Geometry check sheet. Reference: the model listing, model coordinates, mm. A direction names the side the tool comes from. Coordinates: 2 decimals unless noted, no trailing zeros. Loops run counter-clockwise (first coordinate to the right, second up) from the corner with the lowest first, then second, coordinate; pieces in that order, holes last. Notation, with made-up numbers: (-11, 73.25) - (29, 73.25) arc R32 cw to (29, 105.25) - close; hole circle Ø9 at (47.25, 60.25). An arc over 180 degrees is marked (long way). Write item = value, one per line. Start each with the question number.
from build123d import *

# Parameters (mm, degrees)
SKETCH2_W           = 200
SKETCH2_H           = 200
BOSS_EXTRUDE1_DEPTH = 50
SHELL1_T            = -20
CUT_EXTRUDE1_DEPTH  = 50
SKETCH5_R           = 50
BOSS_EXTRUDE2_DEPTH = 28
SKETCH6_R           = 40
CUT_EXTRUDE2_DEPTH  = 34
SKETCH7_R           = 14
CUT_EXTRUDE4_DEPTH  = 46


with BuildPart() as part:
    # Sketch2 → Boss-Extrude1 (new body)
    with BuildSketch(Plane.XY):
        with Locations((-40.678946788, -125.067928938)):
            Rectangle(SKETCH2_W, SKETCH2_H)
    extrude(amount=-BOSS_EXTRUDE1_DEPTH)

    # Shell1
    shell1_openings = [part.faces().sort_by_distance(p)[0] for p in [
        (-40.678946788, -125.067928938, -50),
    ]]
    offset(amount=SHELL1_T, openings=shell1_openings, kind=Kind.INTERSECTION)

    # Sketch3 → Cut-Extrude1 (cut)
    with BuildSketch(Plane.XY):
        Polygon((-13.228603608, -25.067928938), (1.821053212, -51.157579637), (-83.178946788, -51.157579637), (-68.129289968, -25.067928938), align=None)
    extrude(amount=-CUT_EXTRUDE1_DEPTH, mode=Mode.SUBTRACT)

    # Sketch5 → Boss-Extrude2 (add)
    with BuildSketch(Plane(origin=(0, 0, -20), x_dir=(-1, 0, 0), z_dir=(0, 0, -1))):
        with Locations((40.678946788, -125.067928938)):
            Circle(SKETCH5_R)
    extrude(amount=BOSS_EXTRUDE2_DEPTH)

    # Sketch6 → Cut-Extrude2 (cut)
    with BuildSketch(Plane.XY):
        with Locations((-40.678946788, -125.067928938)):
            Circle(SKETCH6_R)
    extrude(amount=-CUT_EXTRUDE2_DEPTH, mode=Mode.SUBTRACT)

    # Sketch7 → Cut-Extrude4 (cut)
    with BuildSketch(Plane(origin=(0, -45.067928938, 0), x_dir=(-1, 0, 0), z_dir=(0, -1, 0))):
        with Locations(Location((40.678946788, 32, 0), (0, 0, 301.002719134))):
            Circle(SKETCH7_R)
    extrude(amount=CUT_EXTRUDE4_DEPTH, mode=Mode.SUBTRACT)


solid = part.part
(1) Sectioned sample at C-C on z = -10.5. Enter the section's corners in (x, y), plus the area to 3 significant figures.
(2) Draft check along Y on faces 5 (the face through (-105, -25.068, -25)), 6 (the face through (-49, -206, -50)), 7 (the face through (-42, -205.068, -35)). Enter one of: pulls with the +Y half, pulls with the -Y half, needs draft (parallel to the pull), parting line crosses it, or undercut.
(3) Sectioned sample at B-B on x = 30.5. Enter the section's corners in (y, z), plus the area to 3 significant figures.
(4) Scan lines: line 1 (Y direction, x = 27.5, z = -30); line 2 (X direction, y = -190.5, z = -42); line 3 (Y direction, x = -69, z = -31). Record each from-to range of solid material in increasing order.
(5) Sectioned sample at A-A on z = -28.5. Enter the section's corners in (x, y).
(6) Sectioned sample at D-D on y = -147. Enter the section's corners in (x, z), plus the area to 3 significant figures.
(7) Depth check by flat-ended pin: pin 1 (10 mm diameter, centred on x = -108, y = -173, fed in from +Z); pin 2 (9.5 mm diameter, centred on x = -38.5, z = -41.5, fed in from +Y). Enter the tip coordinate at first touch or a pass-through.
(8) Tool access check on faces 1 (the face through (-22.221, -160.555, -16.762)), 2 (the face through (39.321, -126, -35)), 3 (the face through (-40, -51.158, -10)), 4 (the face through (-41, -91.068, -40)). Record the directions out of +Z, -Z, +X, -X, +Y, -Y that give a thin tool (end or side, any length) a straight path to the whole face; none if there is none.
Working result:
q1.outline = (-140.68, -225.07) - (59.32, -225.07) - (59.32, -25.07) - (-13.23, -25.07) - (1.82, -51.16) - (-83.18, -51.16) - (-68.13, -25.07) - (-140.68, -25.07) - close; hole circle Ø80 at (-40.68, -125.07)
q1.area = 33,100 mm2
q2.face_5 = pulls with the +Y half
q2.face_6 = needs draft
q2.face_7 = undercut
q3.outline = (-225.07, -50) - (-205.07, -50) - (-205.07, -20) - (-45.07, -20) - (-45.07, -50) - (-25.07, -50) - (-25.07, 0) - (-225.07, 0) - close
q3.area = 5,200 mm2
q4.line_1 = -225.07 to -205.07, -45.07 to -25.07
q4.line_2 = -140.68 to -120.68, 39.32 to 59.32
q4.line_3 = -225.07 to -205.07, -166.27 to -153.32, -96.82 to -83.86, -26.58 to -25.07
q5.outline = (-140.68, -225.07) - (59.32, -225.07) - (59.32, -25.07) - (-13.23, -25.07) - (-1.69, -45.07) - (39.32, -45.07) - (39.32, -205.07) - (-120.68, -205.07) - (-120.68, -45.07) - (-79.67, -45.07) - (-68.13, -25.07) - (-140.68, -25.07) - close; (-54.23, -87.43) - (-54.23, -76.94) arc R50 ccw (long way) to (-27.12, -76.94) - (-27.12, -87.43) arc R40 cw (long way) to start
q6.outline = (-140.68, -50) - (-120.68, -50) - (-120.68, -20) - (-85.61, -20) - (-85.61, -48) - (4.25, -48) - (4.25, -20) - (39.32, -20) - (39.32, -50) - (59.32, -50) - (59.32, 0) - (-7.23, 0) - (-7.23, -34) - (-74.13, -34) - (-74.13, 0) - (-140.68, 0) - close
q6.area = 5,440 mm2
q7.pin_1 = 0
q7.pin_2 = -75.07
q8.face_1 = +Z
q8.face_2 = -Z
q8.face_3 = +Z, -Z
q8.face_4 = +Z, +Y
